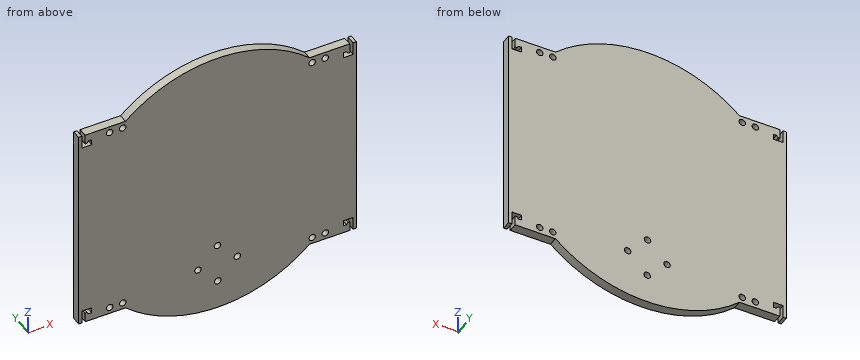
```python
from build123d import *

# Parameters (mm, degrees)
SKETCH4_R           = 2
BOSS_EXTRUDE1_DEPTH = 5.5


with BuildPart() as part:
    # Sketch4 → Boss-Extrude1 (new body)
    with BuildSketch(Plane(origin=(0, 0, 0), x_dir=(1, 0, 0), z_dir=(0, 1, 0))):
        with BuildLine():
            Line((56.335401836, 63.65), (81, 63.65))
            Line((81, 63.65), (81, 57.659411765))
            Line((81, 57.659411765), (80, 57.659411765))
            Line((80, 57.659411765), (79, 58.992745098))
            Line((79, 58.992745098), (77, 58.992745098))
            Line((77, 58.992745098), (77, 55.65))
            Line((77, 55.65), (83, 55.65))
            Line((83, 55.65), (83, 63.65))
            Line((83, 63.65), (85, 63.65))
            Line((85, 63.65), (85, -63.65))
            Line((85, -63.65), (83, -63.65))
            Line((83, -63.65), (83, -55.65))
            Line((83, -55.65), (77, -55.65))
            Line((77, -55.65), (77, -58.992745098))
            Line((77, -58.992745098), (79, -58.992745098))
            Line((79, -58.992745098), (80, -57.659411765))
            Line((80, -57.659411765), (81, -57.659411765))
            Line((81, -57.659411765), (81, -63.65))
            Line((81, -63.65), (56.335401836, -63.65))
            ThreePointArc((56.335401836, -63.65), (0, -85), (-56.335401836, -63.65))
            Line((-56.335401836, -63.65), (-81, -63.65))
            Line((-81, -63.65), (-81, -57.659411765))
            Line((-81, -57.659411765), (-80, -57.659411765))
            Line((-80, -57.659411765), (-79, -58.992745098))
            Line((-79, -58.992745098), (-77, -58.992745098))
            Line((-77, -58.992745098), (-77, -55.65))
            Line((-77, -55.65), (-83, -55.65))
            Line((-83, -55.65), (-83, -63.65))
            Line((-83, -63.65), (-85, -63.65))
            Line((-85, -63.65), (-85, 63.65))
            Line((-85, 63.65), (-83, 63.65))
            Line((-83, 63.65), (-83, 55.65))
            Line((-83, 55.65), (-77, 55.65))
            Line((-77, 55.65), (-77, 58.992745098))
            Line((-77, 58.992745098), (-79, 58.992745098))
            Line((-79, 58.992745098), (-80, 57.659411765))
            Line((-80, 57.659411765), (-81, 57.659411765))
            Line((-81, 57.659411765), (-81, 63.65))
            Line((-81, 63.65), (-56.335401836, 63.65))
            ThreePointArc((-56.335401836, 63.65), (0, 85), (56.335401836, 63.65))
        make_face()
        with Locations(Location((-58, 59.65, 0), (0, 0, 270))):
            Circle(SKETCH4_R, mode=Mode.SUBTRACT)
        with Locations(Location((-66, 59.65, 0), (0, 0, 270))):
            Circle(SKETCH4_R, mode=Mode.SUBTRACT)
        with Locations(Location((66, 59.65, 0), (0, 0, 90))):
            Circle(SKETCH4_R, mode=Mode.SUBTRACT)
        with Locations(Location((58, 59.65, 0), (0, 0, 90))):
            Circle(SKETCH4_R, mode=Mode.SUBTRACT)
        with Locations(Location((66, -59.65, 0), (0, 0, 270))):
            Circle(SKETCH4_R, mode=Mode.SUBTRACT)
        with Locations(Location((58, -59.65, 0), (0, 0, 270))):
            Circle(SKETCH4_R, mode=Mode.SUBTRACT)
        with Locations(Location((-58, -59.65, 0), (0, 0, 90))):
            Circle(SKETCH4_R, mode=Mode.SUBTRACT)
        with Locations(Location((-66, -59.65, 0), (0, 0, 90))):
            Circle(SKETCH4_R, mode=Mode.SUBTRACT)
        with Locations(Location((12.148552835, 54.812479272, 0), (0, 0, 270))):
            Circle(SKETCH4_R, mode=Mode.SUBTRACT)
        with Locations(Location((0, 42.85, 0), (0, 0, 270))):
            Circle(SKETCH4_R, mode=Mode.SUBTRACT)
        with Locations(Location((-11.962479272, 54.998552835, 0), (0, 0, 270))):
            Circle(SKETCH4_R, mode=Mode.SUBTRACT)
        with Locations(Location((0.186073563, 66.961032106, 0), (0, 0, 270))):
            Circle(SKETCH4_R, mode=Mode.SUBTRACT)
    extrude(amount=BOSS_EXTRUDE1_DEPTH)


solid = part.part
```
CAD build for the part. Positions are in the model's coordinates, mm. Give positions to 0.01 mm unless a question says otherwise; leave off trailing zeros. Write each loop counter-clockwise with the first axis right and the second up, starting at its lowest first coordinate (ties: lowest second). Pieces come first, ordered by that corner, then holes. Notation, with made-up numbers: M 75.25,-12.5 L 96.25,-12.5 A21 cw 96.25,12.5 Z; hole C 48.25,42 d4. An arc over 180 degrees is marked long. Return JSON: item names as keys, results as strings. Group by question number.
(1) Band-saw the part on D-D (x = -48). Give the cut face in (y, z), and give its area (3 significant figures).
(2) Flat gauge pins, fed straight in: pin 1 Ø3.5 at (x, z) = (0, -42.85) entering from +Y; pin 2 Ø1 at (x, y) = (-5, 2) entering from +Z; pin 3 Ø2 at (x, y) = (84, 3.5) entering from -Z; pin 4 Ø0.8 at (x, y) = (-80.5, 2) entering from +Z. Where does each tip first touch, or does it go through?
(3) Band-saw the part on A-A (x = -66). Give the cut face in (y, z).
(4) Band-saw the part on C-C (x = 47). Give the cut face in (y, z).
(5) Band-saw the part on B-B (y = 1.6). State how many separate pieces and enclosed holes the cut face has, and give its area (3 significant figures).
(6) Drill centre lines: L1, parallel to X at y = 3.3, z = 63; L2, parallel to Z at x = 58.5, y = 4.75; L3, parallel to X at y = 5.15, z = -43. Where is each one in solid material? Low to high. Write a range as [from, to].
Entries:
{
 "1": {"outline": "M 0,-70.15 L 5.5,-70.15 L 5.5,70.15 L 0,70.15 Z", "area": "772 mm^2"},
 "2": {"pin 1": "passes through", "pin 2": "stops at z = 84.88", "pin 3": "stops at z = -63.65", "pin 4": "stops at z = 63.65"},
 "3": {"outline": "M 0,-63.65 L 5.5,-63.65 L 5.5,-61.65 L 0,-61.65 Z; M 0,-57.65 L 5.5,-57.65 L 5.5,57.65 L 0,57.65 Z; M 0,61.65 L 5.5,61.65 L 5.5,63.65 L 0,63.65 Z"},
 "4": {"outline": "M 0,-70.82 L 5.5,-70.82 L 5.5,70.82 L 0,70.82 Z"},
 "5": {"separate pieces": "1", "enclosed holes": "12", "area": "24,700 mm^2"},
 "6": {"L1": "x = [-85, -83], [-81, 81], [83, 85]", "L2": "z = [-63.65, -61.59], [-57.71, 57.71], [61.59, 63.65]", "L3": "x = [-85, -1.99], [1.99, 85]"}
}
